Can you work these out from the model? Positions are in its coordinate system, mm. A direction names the side the tool comes from. Round coordinates to 2 decimals unless told otherwise and drop trailing zeros. Order: outer loops, then holes, each group sorted by start corner. A loop starts at its lowest first (then second) coordinate and runs counter-clockwise, first axis right, second up. Notation, with made-up numbers: M 70,-6 L 77,-6 A27 ccw 77,21 Z; hole C 53.25,51.5 d11. An arc over 180 degrees is marked long. Answer as a JSON object with one key per item and string values. Group by question number.
from build123d import *

# Parameters (mm, degrees)
SKETCH1_W           = 120
SKETCH1_H           = 220
BOSS_EXTRUDE1_DEPTH = 4
SKETCH2_W           = 120
SKETCH2_H           = 10
BOSS_EXTRUDE2_DEPTH = 40
CUT_EXTRUDE1_START  = -33.5
CUT_EXTRUDE1_DEPTH  = 33.5
BOSS_EXTRUDE3_DEPTH = 20


with BuildPart() as part:
    # Sketch1 → Boss-Extrude1 (new body)
    with BuildSketch(Plane(origin=(0, 0, 0), x_dir=(1, 0, 0), z_dir=(0, 1, 0))):
        Rectangle(SKETCH1_W, SKETCH1_H)
    extrude(amount=BOSS_EXTRUDE1_DEPTH)

    # Sketch2 → Boss-Extrude2 (add)
    with BuildSketch(Plane(origin=(0, 4, 0), x_dir=(1, 0, 0), z_dir=(0, 1, 0))):
        with Locations((0, -105)):
            Rectangle(SKETCH2_W, SKETCH2_H)
    extrude(amount=BOSS_EXTRUDE2_DEPTH)

    # Sketch4 → Cut-Extrude1 (cut)
    with BuildSketch(Plane(origin=(0, 44, 0), x_dir=(1, 0, 0), z_dir=(0, 1, 0)).offset(CUT_EXTRUDE1_START)):
        Polygon((49.06548636, -105), (49.06548636, -102), (45.46548636, -102), (45.46548636, -92), (37.66548636, -92), (37.66548636, -102), (34.06548636, -102), (34.06548636, -105), align=None)
        Polygon((19.35516212, -105), (19.35516212, -102), (15.75516212, -102), (15.75516212, -92), (7.95516212, -92), (7.95516212, -102), (4.35516212, -102), (4.35516212, -105), align=None)
        Polygon((-10.35516212, -105), (-10.35516212, -102), (-13.95516212, -102), (-13.95516212, -92), (-21.75516212, -92), (-21.75516212, -102), (-25.35516212, -102), (-25.35516212, -105), align=None)
    extrude(amount=CUT_EXTRUDE1_DEPTH, mode=Mode.SUBTRACT)

    # Sketch5 → Boss-Extrude3 (add)
    with BuildSketch(Plane(origin=(0, 0, -42.5), x_dir=(-1, 0, 0), z_dir=(0, 0, -1))):
        Polygon((-46.42064848, 4), (-36.71032424, 4), (-36.71032424, 14), (-40.71032424, 14), (-40.71032424, 10.5), (-42.42064848, 10.5), (-42.42064848, 14), (-46.42064848, 14), align=None)
        Polygon((-16.71032424, 4), (-16.71032424, 14), (-12.71032424, 14), (-12.71032424, 10.5), (-11, 10.5), (-11, 14), (-7, 14), (-7, 4), align=None)
        Polygon((13, 4), (13, 14), (17, 14), (17, 10.5), (18.71032424, 10.5), (18.71032424, 14), (22.71032424, 14), (22.71032424, 4), align=None)
    extrude(amount=-BOSS_EXTRUDE3_DEPTH)


solid = part.part
Item 1: On a 3-axis mill with a long thin cutter (end or side, diameter ignored), from which of +Z, -Z, +X, -X, +Y, -Y can I reach the whole of each face in a straight line? I mean faces 4 (the face through (7, 9, -33)), 5 (the face through (12, 9, -22.5)), 6 (the face through (12, 27, 105)), 7 (the face through (-21, 14, -33)), 8 (the face through (-22.71, 9, -33)). Say none if no direction works.
Item 2: Suppose I cut it at A-A, the plane x = -35. Write out the boundary of the cut face in (y, z), and give its area (3 significant figures).
Item 3: Suppose I cut it at C-C, the plane z = 52. Write out the boundary of the cut face in (x, y), and give its area (3 significant figures).
Item 4: I need wall thicknesses on line 1 (Z direction, x = 18.5, y = 21.5); line 2 (Y direction, x = 16, z = 68.5); line 3 (Z direction, x = -43.5, y = 17). Which ranges of each line are inside material? Lowest first, please.
Item 5: If we mould it in two halves opening along Z, with no side actions, what happens to faces 1 (the face through (39, 14, -33)), 2 (the face through (41, 27, 105)), 3 (the face through (12, 9, -42.5))? For each: +Z half, -Z half, draft (parallel to the pull), parting line (faces both ways), or undercut.
Item 6: Suppose I cut it at B-B, the plane y = 32.5. Write out the boundary of the cut face in (x, z).
Item 7: I'm going to push flat-ended pins straight in: pin 1 Ø10 at (x, y) = (46.5, 22.5) entering from -Z; pin 2 Ø6 at (x, z) = (25, 87.5) entering from +Y; pin 3 Ø1.8 at (y, z) = (11.5, -27.5) entering from +X. Where does each tip first touch, or does it pass through?
Computed:
{
 "1": {"face 4": "-Z, +Y", "face 5": "+X, -X, +Y", "face 6": "+Y", "face 7": "-Z, +X, -X, +Y", "face 8": "-Z, -X, +Y"},
 "2": {"outline": "M 0,-110 L 4,-110 L 4,100 L 44,100 L 44,110 L 0,110 Z", "area": "1,280 mm^2"},
 "3": {"outline": "M -60,0 L 60,0 L 60,4 L -60,4 Z", "area": "480 mm^2"},
 "4": {"line 1": "z = 100 to 102, 105 to 110", "line 2": "y = 0 to 4", "line 3": "z = 100 to 110"},
 "5": {"face 1": "draft", "face 2": "undercut", "face 3": "-Z half"},
 "6": {"outline": "M -60,100 L -21.76,100 L -21.76,102 L -25.36,102 L -25.36,105 L -10.36,105 L -10.36,102 L -13.96,102 L -13.96,100 L 7.96,100 L 7.96,102 L 4.36,102 L 4.36,105 L 19.36,105 L 19.36,102 L 15.76,102 L 15.76,100 L 37.67,100 L 37.67,102 L 34.07,102 L 34.07,105 L 49.07,105 L 49.07,102 L 45.47,102 L 45.47,100 L 60,100 L 60,110 L -60,110 Z"},
 "7": {"pin 1": "stops at z = 100", "pin 2": "stops at y = 4", "pin 3": "stops at x = 46.42"}
}
